Part print with two shaded views. Sizes in mm from the minimum x, y, z corner. A direction names the side the tool comes from. Give positions to 0.01 mm unless a question says otherwise; leave off trailing zeros. Loops run counter-clockwise (first coordinate to the right, second up) from the corner with the lowest first, then second, coordinate; pieces in that order, holes last. Notation, with made-up numbers: (43.25, -18.75) -> (55.25, -18.75) arc R14 cw to (55.25, 5.25) -> close; hole circle Ø3 at (36, 18). An arc over 180 degrees is marked (long way). One line per question, with ' | ' between items. Start each with the question number.
(1) Slice it at C-C, the plane y = 89. Write the cut outline in (x, z) (3 decimals).
(2) Mould opens along Z. For the marked faces 1, 2, 3 and 4 say: pulls with the +Z half, pulls with the -Z half, needs draft (parallel to the pull), parting line crosses it, or undercut.
(3) 3-axis set-ups, long thin cutter, end or side, ignore diameter. For the marked faces 5 and 6: which of +Z, -Z, +X, -X, +Y, -Y reach the whole face in a straight line?
(4) Slice it at D-D, the plane y = 58. Write the cut outline in (x, z) (1 decimal).
(5) Slice it at A-A, the plane x = 43. Write the cut outline in (y, z) (3 decimals), then the cut area to 3 significant figures.
(6) Drill centre lines: L1, parallel to Z at x = 23, y = 75 (3 decimals); L2, parallel to X at y = 34, z = 23 (3 decimals); L3, parallel to Y at x = 3, z = 21. Where is each one in solid material? Low to high. Write a range as from..to.
(7) Flat gauge pins, fed straight in: pin 1 Ø1 at (y, z) = (89, 1.5) entering from +X; pin 2 Ø4 at (x, z) = (46.5, 14) entering from +Y; pin 3 Ø10 at (x, z) = (33, 19) entering from -Y. Where does each tip first touch, or does it go through?
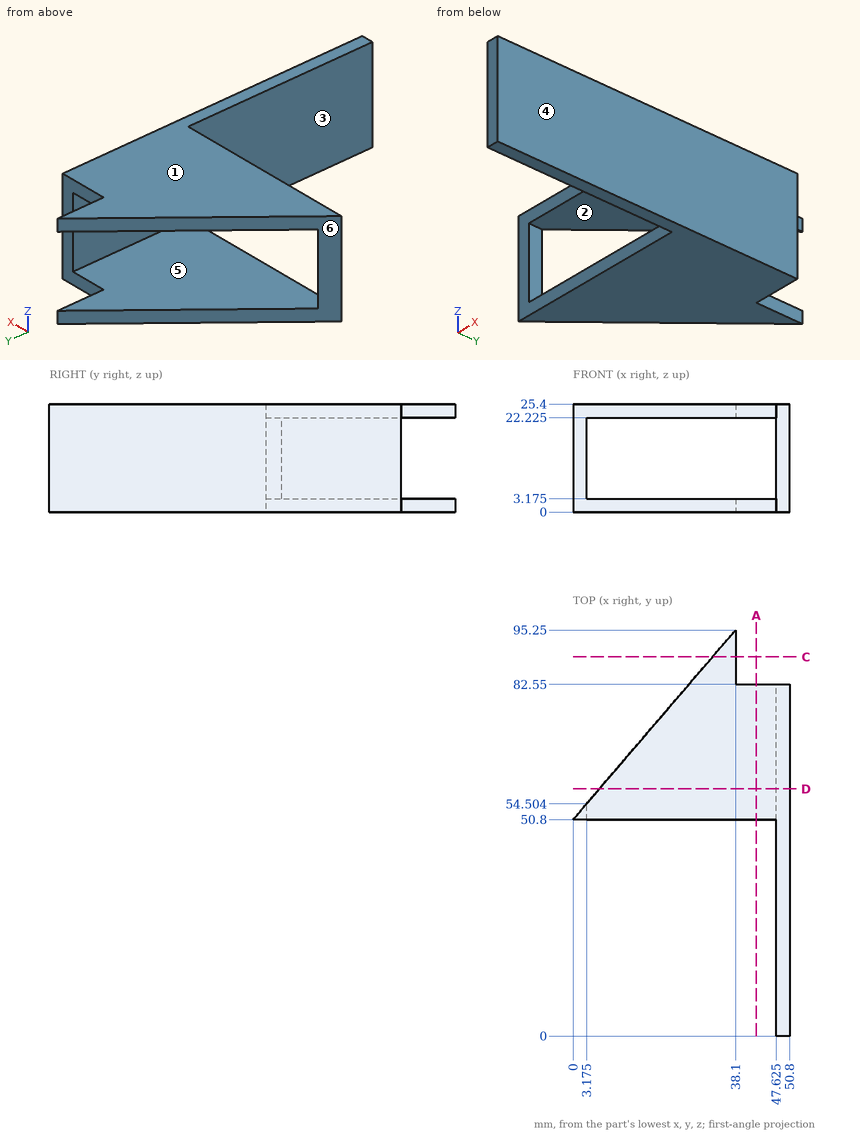
Final values:
1) outline: (32.743, 0) -> (38.1, 0) -> (38.1, 3.175) -> (32.743, 3.175) -> close; (32.743, 22.225) -> (38.1, 22.225) -> (38.1, 25.4) -> (32.743, 25.4) -> close
2) face 1: pulls with the +Z half | face 2: undercut | face 3: undercut | face 4: needs draft
3) face 5: +Y, -Y | face 6: +Z, -Z, -X, +Y
4) outline: (6.2, 0) -> (50.8, 0) -> (50.8, 25.4) -> (6.2, 25.4) -> (6.2, 22.2) -> (47.6, 22.2) -> (47.6, 3.2) -> (6.2, 3.2) -> close
5) outline: (50.8, 0) -> (82.55, 0) -> (82.55, 3.175) -> (50.8, 3.175) -> close; (50.8, 22.225) -> (82.55, 22.225) -> (82.55, 25.4) -> (50.8, 25.4) -> close | area: 202 mm2
6) L1: 0..3.175, 22.225..25.4 | L2: 47.625..50.8 | L3: 50.8..54.3
7) pin 1: x = 38.1 | pin 2: y = 82.55 | pin 3: y = 50.8
